```python
from build123d import *

# Parameters (mm, degrees)
BOSS_EXTRUDE1_DEPTH = 38.1
SKETCH2_W           = 31.75
SKETCH2_H           = 31.75
CUT_EXTRUDE1_DEPTH  = 206.593204132


with BuildPart() as part:
    # Sketch1 → Boss-Extrude1 (new body)
    with BuildSketch(Plane(origin=(0, 0, 0), x_dir=(0, 0, -1), z_dir=(1, 0, 0))):
        with BuildLine():
            Line((168.785784374, 0), (198.40702, 38.1))
            Line((198.40702, 38.1), (14.810617813, 38.1))
            ThreePointArc((14.810617813, 38.1), (21.675298243, 29.653694926), (24.13, 19.05))
            ThreePointArc((24.13, 19.05), (21.675298243, 8.446305074), (14.810617813, 0))
            Line((14.810617813, 0), (168.785784374, 0))
        make_face()
    extrude(amount=BOSS_EXTRUDE1_DEPTH)

    # Sketch2 → Cut-Extrude1 (cut, through all)
    with BuildSketch(Plane.XY):
        with Locations((19.05, 19.05)):
            Rectangle(SKETCH2_W, SKETCH2_H)
    extrude(amount=-CUT_EXTRUDE1_DEPTH, mode=Mode.SUBTRACT)


solid = part.part
```
Verification items for the finished model (mm, model axes). A direction names the side the tool comes from. Coordinates: 2 decimals unless noted, no trailing zeros. Loops run counter-clockwise (first coordinate to the right, second up) from the corner with the lowest first, then second, coordinate; pieces in that order, holes last. Notation, with made-up numbers: (31, -38.75) - (71, -38.75) arc R12 ccw to (71, -25.75) - close; hole circle Ø7 at (56.25, 25). An arc over 180 degrees is marked (long way). Put each result on its own line as item: value.
Item 1: Section check A-A (x = 19.5). Enter the section's corners in (y, z) (3 decimals), then the cut area to 3 significant figures.
Conclusion:
outline: (0, -168.786) - (3.175, -171.254) - (3.175, -18.173) arc R24.13 cw to (0, -14.811) - close; (34.925, -195.939) - (38.1, -198.407) - (38.1, -14.811) arc R24.13 cw to (34.925, -18.173) - close
area: 1,060 mm2
Item 2: Draft check along Y on faces 1 (the face through (38.1, 19, -105)), 2 (the face through (19, 0, -91)), 3 (the face through (19, 3.175, -94)). Enter one of: pulls with the +Y half, pulls with the -Y half, needs draft (parallel to the pull), parting line crosses it, or undercut.
Conclusion:
face 1: needs draft
face 2: pulls with the -Y half
face 3: undercut
Item 3: Scan lines: line 1 along X through (y, z) = (13, -50) (3 decimals); line 2 along Y through (x, z) = (14, -175) (3 decimals). Record each from-to range of solid material in increasing order.
Conclusion:
line 1: x = 0 to 3.175, 34.925 to 38.1
line 2: y = 34.925 to 38.1
Item 4: Section check C-C (z = -88). Enter the section's corners in (x, y) (3 decimals), then the cut area to 3 significant figures.
Conclusion:
outline: (0, 0) - (38.1, 0) - (38.1, 38.1) - (0, 38.1) - close; hole (3.175, 3.175) - (34.925, 3.175) - (34.925, 34.925) - (3.175, 34.925) - close
area: 444 mm2
Item 5: Section check B-B (y = 7). Enter the section's corners in (x, z) (3 decimals).
Conclusion:
outline: (0, -174.228) - (3.175, -174.228) - (3.175, -20.906) - (0, -20.906) - close; (34.925, -174.228) - (38.1, -174.228) - (38.1, -20.906) - (34.925, -20.906) - close
Item 6: Gauge pin test, flat end, axial feed: pin 1 Ø16 at (x, z) = (22, -87.5) entering from -Y. Record the tip position at first contact, or that the pin passes through.
Conclusion:
pin 1: stops at y = 0
Item 7: Set-up check for faces 4 (the face through (0, 19, -105)), 5 (the face through (19, 34.925, -106)): record each of +Z, -Z, +X, -X, +Y, -Y from which the full face is reachable in a straight line by a thin tool's end or side.
Conclusion:
face 4: +Z, -Z, -X, +Y, -Y
face 5: +Z, -Z
